Answer from the drawing. Dimensions are ordinates in mm from the lowest x, y and z of the part. A direction names the side the tool comes from. Coordinates: 2 decimals unless noted, no trailing zeros. Order: outer loops, then holes, each group sorted by start corner. A loop starts at its lowest first (then second) coordinate and runs counter-clockwise, first axis right, second up. Notation, with made-up numbers: (24, 47.5) -> (65, 47.5) arc R16 ccw to (65, 74.5) -> close; hole circle Ø10 at (-31, 40). An arc over 180 degrees is marked (long way). Answer in a Markdown table with one row per item.
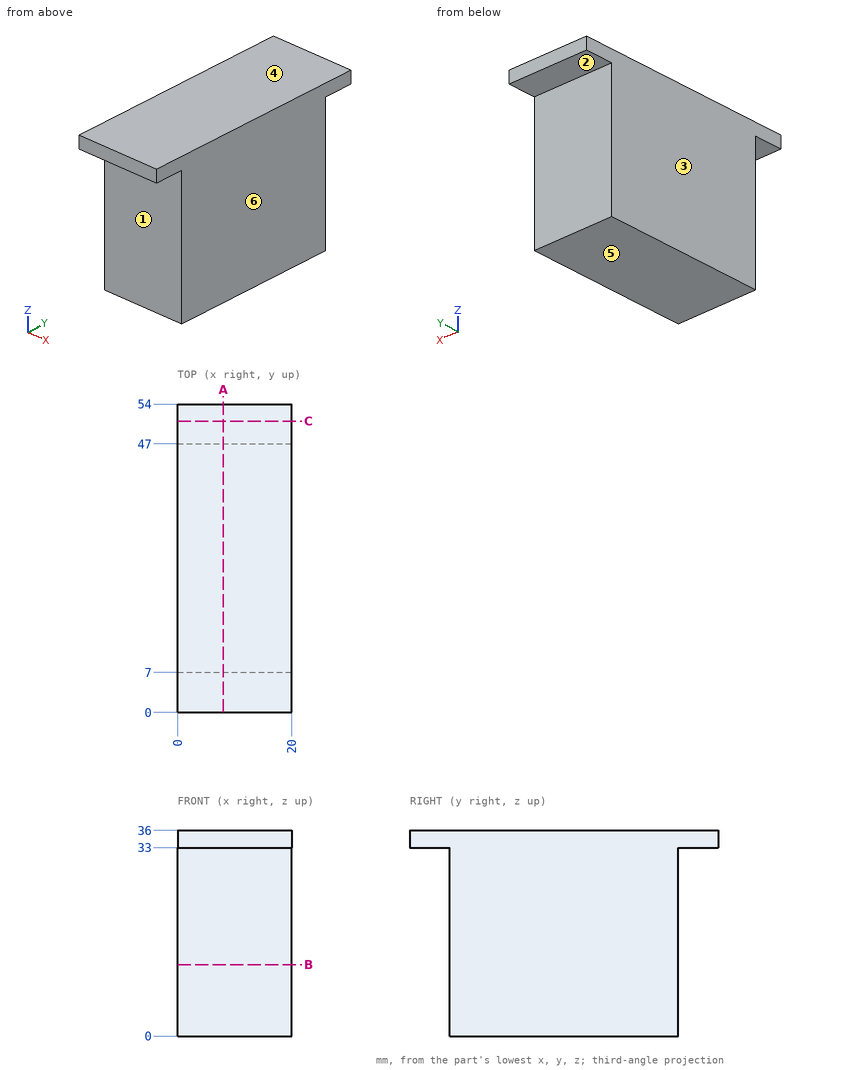
(1) Flat-ended cylindrical pins translate along their axes: pin 1 (2 mm diameter, centred on x = 14, y = 2, fed in from -Z); pin 2 (6 mm diameter, centred on x = 3.5, z = 15, fed in from +Y). Find the tip coordinate at first contact, or state that the pin passes through.
Check values:
| item | result |
|---|---|
| pin 1 | z = 33 |
| pin 2 | y = 47 |
(2) Find the intervals of material crossed by line 1 along Y through (x, z) = (19.25, 17); line 2 along Z through (x, y) = (15, 4), in increasing order. Write a range as from..to.
Check values:
| item | result |
|---|---|
| line 1 | 7..47 |
| line 2 | 33..36 |
(3) A cutting plane is placed at C-C, the plane y = 51. Determine the outline of the cut face in (x, z).
Check values:
| item | result |
|---|---|
| outline | (0, 33) -> (20, 33) -> (20, 36) -> (0, 36) -> close |
(4) A cutting plane is placed at B-B, the plane z = 12.5. Determine the outline of the cut face in (x, y), then the cut area to 3 significant figures.
Check values:
| item | result |
|---|---|
| outline | (0, 7) -> (20, 7) -> (20, 47) -> (0, 47) -> close |
| area | 800 mm² |
(5) A cutting plane is placed at A-A, the plane x = 8. Determine the outline of the cut face in (y, z).
Check values:
| item | result |
|---|---|
| outline | (0, 33) -> (7, 33) -> (7, 0) -> (47, 0) -> (47, 33) -> (54, 33) -> (54, 36) -> (0, 36) -> close |
(6) For a pull along Z with two mould halves and no side action, classify the marked faces 4, 5 and 6 as released by +Z, released by -Z, zero draft, split by the parting line, or undercut.
Check values:
| item | result |
|---|---|
| face 4 | released by +Z |
| face 5 | released by -Z |
| face 6 | zero draft |
(7) Which of the six approach directions +Z, -Z, +X, -X, +Y, -Y give full straight-line access (tool end or side, diameter ignored) to the marked faces 1, 2 and 3?
Check values:
| item | result |
|---|---|
| face 1 | -Z, +X, -X, -Y |
| face 2 | -Z, +X, -X, +Y |
| face 3 | +Z, -Z, -X, +Y, -Y |
